```python
from build123d import *

# Parameters (mm, degrees)
BOSS_EXTRU_1_DEPTH = 3


with BuildPart() as part:
    # Esquisse1 → Boss.-Extru.1 (new body)
    with BuildSketch(Plane(origin=(0, 0, 0), x_dir=(1, 0, 0), z_dir=(0, 1, 0))):
        Polygon((0, 32), (0, 17.5), (80, 17.5), (80, 32), (74.3, 32), (74.3, 35), (65.7, 35), (65.7, 32), (54.3, 32), (54.3, 35), (45.7, 35), (45.7, 32), (34.3, 32), (34.3, 35), (25.7, 35), (25.7, 32), (14.3, 32), (14.3, 35), (5.7, 35), (5.7, 32), align=None)
        Polygon((25.7, 3), (25.7, 0), (34.3, 0), (34.3, 3), (45.7, 3), (45.7, 0), (54.3, 0), (54.3, 3), (65.7, 3), (65.7, 0), (74.3, 0), (74.3, 3), (80, 3), (80, 17.5), (0, 17.5), (0, 3), (5.7, 3), (5.7, 0), (14.3, 0), (14.3, 3), (20, 3), align=None)
    extrude(amount=BOSS_EXTRU_1_DEPTH)


solid = part.part
```
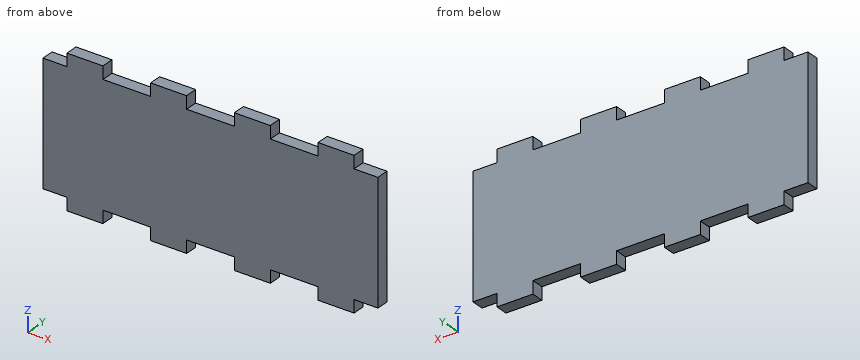
Here's how the part is built. I have some questions about the finished solid (model axes, mm). Give positions to 0.01 mm unless a question says otherwise; leave off trailing zeros. Order: outer loops, then holes, each group sorted by start corner. A loop starts at its lowest first (then second) coordinate and runs counter-clockwise, first axis right, second up. Notation, with made-up numbers: M 26.25,-16.5 L 71.25,-16.5 A13 ccw 71.25,-6.5 Z; hole C -0.75,12 d6. An arc over 180 degrees is marked long. Use a Markdown table: item, result. Add a question column.
1. Suppose I cut it at A-A (x = 56). List the corners of the cut face in (y, z) for me.
2. I need wall thicknesses on probe 1 along Z at (x, y) = (43, 1.85). Which ranges of the line are inside material? Lowest first, please. Write a range as from..to.
3. For pin 1 Ø0.9 at (y, z) = (2, -2) entering from +X; pin 2 Ø0.9 at (y, z) = (1.5, -1) entering from -X; pin 3 Ø0.9 at (x, y) = (76, 2) entering from -Z, each with a flat end and sliding along its axis, tell me the tip position at first contact or that it passes through.
Results list:
| question | item | result |
|---|---|---|
| 1 | outline | M 0,-32 L 3,-32 L 3,-3 L 0,-3 Z |
| 2 | probe 1 | z = -32..-3 |
| 3 | pin 1 | stops at x = 74.3 |
| 3 | pin 2 | stops at x = 5.7 |
| 3 | pin 3 | stops at z = -32 |
